```python
from build123d import *

# Parameters (mm, degrees)
F0_R         = 8.75
F4_R         = 3
F6_DEPTH     = 10
F10_R        = 9
F5_FACE1_R   = 3
F12_DEPTH    = 10
F13_T        = 1
F13_T4_ANGLE = 180.000000001
F13_T6_ANGLE = 180.000000001


# Not quite as in the source:
# - a shell that OpenCascade refuses in one call is made with other operations: the cavity is built on its own and cut out


with BuildPart() as f5:
    # F0 (on Front) → F5 section 0
    with BuildSketch(Plane.XZ):
        Circle(F0_R)
    # F4 (on line) → F5 section 1
    with BuildSketch(Plane(origin=(0, 15, 0), x_dir=(-1, 0, 0), z_dir=(0, 1, 0))):
        Circle(F4_R)
    loft()

    # F6 (add): a face of the model
    f6_faces = [f5.faces().sort_by_distance(p)[0] for p in [
        (0, 0, 0),
    ]]
    extrude(f6_faces, amount=F6_DEPTH)

    # F10 (on line) → F11 section 0
    with BuildSketch(Plane(origin=(0, 20, 0), x_dir=(-1, 0, 0), z_dir=(0, 1, 0))):
        Circle(F10_R)
    # F5_face1 (on face) → F11 section 1
    with BuildSketch(Plane(origin=(0, 15, 0), x_dir=(-1, 0, 0), z_dir=(0, 1, 0))):
        Circle(F5_FACE1_R)
    loft()

    # F12 (add): a face of the model
    f12_faces = [f5.faces().sort_by_distance(p)[0] for p in [
        (0, 20, 0),
    ]]
    extrude(f12_faces, amount=F12_DEPTH)

    # F13: shell of thickness 1, made by hand


with BuildPart() as f13_core1:
    # F13_t2: copy of F5
    add(f5.part)

    # the walls: a layer under each face that stays
    f13_faces = [f13_core1.faces().sort_by_distance(p)[0] for p in [
        (-5.875, 7.5, 0),
        (6, 17.5, 0),
        (-8.75, -5, 0),
        (9, 25, 0),
    ]]
    thicken(f13_faces, amount=-F13_T, mode=Mode.SUBTRACT)

    # F13_s3 → F13_t4 (revolve, cut)
    with BuildSketch(Plane.XY):
        Polygon((3.0157393052, 14.9958971473), (2.0662538827, 14.6420639884), (1.8101483908, 15.3101652716), (2.3598156003, 15.7682212796), align=None)
    revolve(axis=Axis((0, 15, 0), (0, -1, 0)), revolution_arc=F13_T4_ANGLE, mode=Mode.SUBTRACT)

    # F13_s5 → F13_t6 (revolve, cut)
    with BuildSketch(Plane.XY):
        Polygon((-3.0157393052, 14.9958971473), (-2.0662538827, 14.6420639884), (-1.8101483908, 15.3101652716), (-2.3598156003, 15.7682212796), align=None)
    revolve(axis=Axis((0, 15, 0), (0, -1, 0)), revolution_arc=F13_T6_ANGLE, mode=Mode.SUBTRACT)


with BuildPart() as f5_1:
    add(f5.part)

    # what is left inside the walls is the cavity
    f13_cavity = [f13_core1.part.solids().sort_by_distance(p)[0] for p in [
        (-5.84608, 4.753709, 0),
    ]]
    add(f13_cavity, mode=Mode.SUBTRACT)


solid = f5_1.part
```
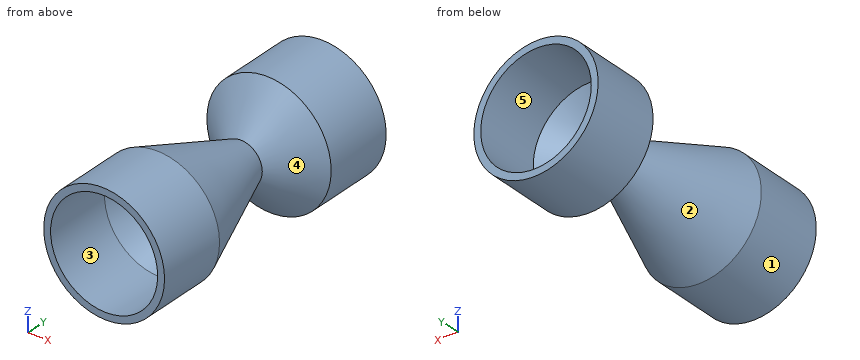
Input: part model. Units: mm. Frame: model coordinates. Face numbers are marked on the shaded views. A direction names the side the tool comes from. Give positions to 0.01 mm unless a question says otherwise; leave off trailing zeros. Order: outer loops, then holes, each group sorted by start corner. A loop starts at its lowest first (then second) coordinate and runs counter-clockwise, first axis right, second up. Notation, with made-up numbers: M -23,-7 L 22,-7 A21 cw 22,2 Z; hole C -20,-29.5 d7. An arc over 180 degrees is marked long. Return JSON: item names as keys, results as strings.
Item 1: First-contact query: P1, Ø6, axis at x = -6, y = -2.5, coming from the -Z side; P2, Ø2, axis at x = -1.5, y = 21.5, coming from the -Z side; P3, Ø5, axis at x = -3.5, z = -1.5, coming from the +Y side. Flat tips, straight axial feed; report the tip coordinate or a pass-through.
Solutions:
{"P1": "z = -8.22", "P2": "z = -8.99", "P3": "y = 19.06"}
Item 2: Pull-direction query (Y, two-part tool) for the marked faces 1 and 2; classes: +Y half, -Y half, draft (parallel to the pull), parting line (faces both ways), or undercut.
Solutions:
{"face 1": "draft", "face 2": "undercut"}
Item 3: Access query for the marked faces 3, 4 and 5. Directions: +Z, -Z, +X, -X, +Y, -Y. A direction counts if a zero-diameter tool reaches every point of the face in a straight line with its end or side. Return the directions, or none.
Solutions:
{"face 3": "-Y", "face 4": "none", "face 5": "+Y"}
Item 4: Cut plane B-B (y = 3.5). Return loops of the section in (x, z).
Solutions:
{"outline": "C 0,0 d14.82; hole C 0,0 d12.67"}
Item 5: Ray query, probe 1 along Z at (x, y) = (0, 27.75); probe 2 along X at (y, z) = (-5.5, 0). Return the intervals inside material, ascending.
Solutions:
{"probe 1": "-9 to -8, 8 to 9", "probe 2": "-8.75 to -7.75, 7.75 to 8.75"}
Item 6: Cut plane A-A (y = -7). Return loops of the section in (x, z).
Solutions:
{"outline": "C 0,0 d17.5; hole C 0,0 d15.5"}
